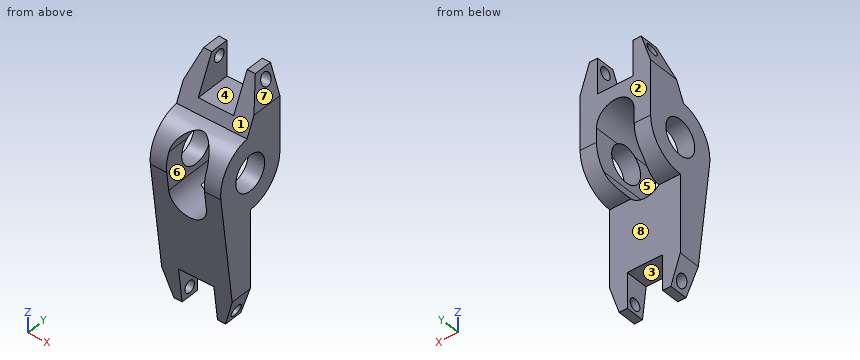
from build123d import *
from OCP.BRepFilletAPI import BRepFilletAPI_MakeChamfer

# Parameters (mm, degrees)
SKETCH2_R               = 4.765
BOSS_EXTRUDE1_DEPTH     = 9.5
CHAMFER1_SIZE           = 2.54
CHAMFER1_SIZE2          = 7.62
CHAMFER2_SIZE           = 7.62
CHAMFER2_SIZE2          = 2.54
CUT_EXTRUDE1_DEPTH      = 41.693294902
CUT_EXTRUDE1_DEPTH_BACK = 41.693294902
CUT_EXTRUDE2_DEPTH      = 41.69329495
CUT_EXTRUDE2_DEPTH_BACK = 41.69329495
SKETCH4_W               = 9.53
SKETCH4_H               = 9.53
CUT_EXTRUDE3_DEPTH      = 41.69329495
CUT_EXTRUDE3_DEPTH_BACK = 41.69329495
SKETCH5_R               = 1.59


with BuildPart() as part:
    # Sketch2 → Boss-Extrude1 (new, symmetric)
    with BuildSketch(Plane(origin=(0, 0, 0), x_dir=(0, 0, -1), z_dir=(1, 0, 0))):
        with BuildLine():
            Line((0, 9.765), (-22.225, 9.765))
            Line((-22.225, 9.765), (-22.225, 4.765))
            Line((-22.225, 4.765), (-9.705896356, -1.072753903))
            ThreePointArc((-9.705896356, -1.072753903), (-6.045130296, -7.668873758), (1.223496761, -9.688048342))
            Line((1.223496761, -9.688048342), (38.345, -5))
            Line((38.345, -5), (38.345, 0))
            Line((38.345, 0), (9.765, 0))
            ThreePointArc((9.765, 0), (6.904897718, 6.904897718), (0, 9.765))
        make_face()
        Circle(SKETCH2_R, mode=Mode.SUBTRACT)
    extrude(amount=BOSS_EXTRUDE1_DEPTH, both=True)

    # Chamfer1: one chamfer whose edges measure the first distance from different faces: ONE call of the kernel's chamfer builder (chamfer() names one face for all edges)
    chamfer1_edges_1 = [part.edges().sort_by_distance(p)[0] for p in [
        (9.5, 7.265, 22.225),
    ]]
    chamfer1_side_1 = [part.faces().sort_by_distance(p)[0] for p in [
        (0, 7.265, 22.225),
    ]]
    chamfer1_edges_2 = [part.edges().sort_by_distance(p)[0] for p in [
        (9.5, -2.5, -38.345),
    ]]
    chamfer1_side_2 = [part.faces().sort_by_distance(p)[0] for p in [
        (0, -2.5, -38.345),
    ]]
    chamfer1 = BRepFilletAPI_MakeChamfer(part.part.solid().wrapped)
    for e in chamfer1_edges_1:
        chamfer1.Add(CHAMFER1_SIZE, CHAMFER1_SIZE2, e.wrapped, chamfer1_side_1[0].wrapped)  # the first distance lies on this face
    for e in chamfer1_edges_2:
        chamfer1.Add(CHAMFER1_SIZE, CHAMFER1_SIZE2, e.wrapped, chamfer1_side_2[0].wrapped)  # the first distance lies on this face
    add(Compound.cast(chamfer1.Shape()), mode=Mode.REPLACE)

    # Chamfer2
    chamfer2_edges = [part.edges().sort_by_distance(p)[0] for p in [
        (-9.5, -2.5, -38.345),
        (-9.5, 7.265, 22.225),
    ]]
    chamfer2_side = [part.faces().sort_by_distance(p)[0] for p in [
        (-9.5, -0.130280991, -5.201405079),
    ]]
    chamfer(chamfer2_edges, length=CHAMFER2_SIZE, length2=CHAMFER2_SIZE2, reference=chamfer2_side[0])

    # Sketch3 → Cut-Extrude1 (cut, two sides: drawn at the far end of the back side and taken through both)
    with BuildSketch(Plane(origin=(0, 0, 0), x_dir=(1, 0, 0), z_dir=(0, 1, 0)).offset(-CUT_EXTRUDE1_DEPTH_BACK)):
        with BuildLine():
            Line((-5.08, -3.81), (-5.08, 6.35))
            ThreePointArc((-5.08, 6.35), (0, 11.43), (5.08, 6.35))
            Line((5.08, 6.35), (5.08, -3.81))
            ThreePointArc((5.08, -3.81), (0, -8.89), (-5.08, -3.81))
        make_face()
    extrude(amount=CUT_EXTRUDE1_DEPTH + CUT_EXTRUDE1_DEPTH_BACK, mode=Mode.SUBTRACT)

    # Sketch4 → Cut-Extrude2 (cut, two sides: drawn at the far end of the back side and taken through both)
    with BuildSketch(Plane(origin=(0, 0, 0), x_dir=(1, 0, 0), z_dir=(0, 1, 0)).offset(-CUT_EXTRUDE2_DEPTH_BACK)):
        with Locations((0, 33.58)):
            Rectangle(SKETCH4_W, SKETCH4_H)
        with Locations((0, -17.46)):
            Rectangle(SKETCH4_W, SKETCH4_H)
    extrude(amount=CUT_EXTRUDE2_DEPTH + CUT_EXTRUDE2_DEPTH_BACK, mode=Mode.SUBTRACT)

    # Sketch5 → Cut-Extrude3 (cut, two sides: drawn at the far end of the back side and taken through both)
    with BuildSketch(Plane(origin=(0, 0, 0), x_dir=(0, 0, -1), z_dir=(1, 0, 0)).offset(-CUT_EXTRUDE3_DEPTH_BACK)):
        with Locations((35.805, -2.54)):
            Circle(SKETCH5_R)
        with Locations(Location((-19.685, 7.225, 0), (0, 0, 180))):
            Circle(SKETCH5_R)
    extrude(amount=CUT_EXTRUDE3_DEPTH + CUT_EXTRUDE3_DEPTH_BACK, mode=Mode.SUBTRACT)


solid = part.part
Part model, mm, in its own coordinate system. Face numbers are marked on the shaded views. A direction names the side the tool comes from. Coordinates: 2 decimals unless noted, no trailing zeros. Loops run counter-clockwise (first coordinate to the right, second up) from the corner with the lowest first, then second, coordinate; pieces in that order, holes last. Notation, with made-up numbers: M 2,14.5 L 45,14.5 A20 cw 45,37.5 Z; hole C -20.75,85 d1. An arc over 180 degrees is marked long. Use a Markdown table: item, result. Add a question column.
Q1. Cut at B-B (z = -35). Write the cut outline in (x, y) (3 decimals), and give its area (3 significant figures).
Q2. Which spindle directions (+Z, -Z, +X, -X, +Y, -Y) get a long thin tool onto all of the face, cutting with end or side? Do the marked faces 1, 2, 3, 4 and 5. Say none if no direction does.
Q3. Cut at D-D (z = -13.5). Write the cut outline in (x, y), and give its area (3 significant figures).
Q4. Probe L1, parallel to Z at x = 5.9, y = -2.54 (3 decimals); L2, parallel to Y at x = 8.3, z = 0 (3 decimals); L3, parallel to Z at x = -7.5, y = -2.54 (3 decimals). List the from-to ranges inside material, lowest first.
Q5. Cut at A-A (x = 1.5). Write the cut outline in (y, z) (1 decimal).
Q6. Pin check, flat tips, straight feed: P1, Ø3, axis at x = -2, z = -24.5, coming from the -Y side; P2, Ø5, axis at y = -2, z = -35.5, coming from the +X side; P3, Ø4, axis at y = 7.225, z = 19.685, coming from the -X side. Stop position of each tip, or through.
Q7. Mould opens along X. For the marked faces 6, 7 and 8 say: +X half, -X half, draft (parallel to the pull), parting line (faces both ways), or undercut.
Q8. Cut at C-C (x = -6). Write the cut outline in (y, z) (1 decimal).
Worked out:
| question | item | result |
|---|---|---|
| 1 | outline | M -8.075,-5.422 L -4.765,-5.422 L -4.765,-3.911 L -8.075,-3.911 Z; M -8.075,-1.169 L -4.765,-1.169 L -4.765,0 L -8.075,0 Z; M 4.765,-5.422 L 8.075,-5.422 L 8.075,-3.911 L 4.765,-3.911 Z; M 4.765,-1.169 L 8.075,-1.169 L 8.075,0 L 4.765,0 Z |
| 1 | area | 17.7 mm2 |
| 2 | face 1 | +Z, +X, -X, -Y |
| 2 | face 2 | +Z, -Z, +X, -X, +Y |
| 2 | face 3 | -Z, +Y, -Y |
| 2 | face 4 | +Z, +Y, -Y |
| 2 | face 5 | +Y, -Y |
| 3 | outline | M -9.5,-8.14 L 9.5,-8.14 L 9.5,0 L -9.5,0 Z |
| 3 | area | 155 mm2 |
| 4 | L1 | z = -38.345 to -37.395, -34.215 to -4.032, 4.032 to 9.429 |
| 4 | L2 | y = -9.765 to -4.765, 4.765 to 9.765 |
| 4 | L3 | z = -34.215 to -4.032, 4.032 to 9.429 |
| 5 | outline | M -8.4,-11.2 L -6.2,-28.8 L 0,-28.8 L 0,-11.2 Z; M -4.5,8.7 L 9.8,8.7 L 9.8,12.7 L 0.3,12.7 L -1.1,9.7 A9.8 ccw Z |
| 6 | P1 | stops at y = -6.94 |
| 6 | P2 | stops at x = 8.74 |
| 6 | P3 | stops at x = -8.47 |
| 7 | face 6 | undercut |
| 7 | face 7 | +X half |
| 7 | face 8 | draft |
| 8 | outline | M -9.7,-1.2 L -5,-38.3 L 0,-38.3 L 0,-9.8 A9.8 ccw 9.8,0 L 9.8,22.2 L 4.8,22.2 L -1.1,9.7 A9.8 ccw Z; hole C 0,0 d9.5; hole C -2.5,-35.8 d3.2; hole C 7.2,19.7 d3.2 |
